For this review, take the finished solid that the model builds, in its own axes (mm). Round coordinates to 2 decimals unless told otherwise and drop trailing zeros. Order: outer loops, then holes, each group sorted by start corner. A loop starts at its lowest first (then second) coordinate and runs counter-clockwise, first axis right, second up. Notation, with made-up numbers: M -1,-21 L 29,-21 A27 cw 29,16 Z; hole C 9,88 d3. An arc over 180 degrees is marked long. Put each result on its own line as item: value.
from build123d import *

# Parameters (mm, degrees)
BOSS_EXTRUDE2_DEPTH   = 25.4
F_8_CLEARANCE_HOLE1_D = 4.191
FILLET1_R             = 2.54


with BuildPart() as part:
    # Sketch2 → Boss-Extrude2 (new body)
    with BuildSketch(Plane.XY):
        Polygon((92.922616299, 8.043671593), (48.599616303, 8.043671593), (48.599616303, 260.300358649), (92.922616299, 69.957537027), align=None)
    extrude(amount=BOSS_EXTRUDE2_DEPTH)

    # #8 Clearance Hole1 (through all)
    with Locations(Plane(origin=(0, 0, 0), x_dir=(-1, 0, 0), z_dir=(0, 0, -1))):
        with Locations((-80.22261633, 20.616671539), (-67.52261633, 20.616671539), (-54.82261633, 20.616671539)):
            Hole(F_8_CLEARANCE_HOLE1_D / 2)

    # Fillet1
    fillet1_edges = [part.edges().sort_by_distance(p)[0] for p in [
        (92.922616299, 39.00060431, 25.4),
        (70.761116301, 165.128947838, 25.4),
        (48.599616303, 134.172015121, 25.4),
        (70.761116301, 165.128947838, 0),
        (92.922616299, 39.00060431, 0),
        (70.761116301, 8.043671593, 0),
        (48.599616303, 134.172015121, 0),
        (70.761116301, 8.043671593, 25.4),
        (48.599616303, 260.300358649, 12.7),
        (92.922616299, 69.957537027, 12.7),
        (92.922616299, 8.043671593, 12.7),
        (48.599616303, 8.043671593, 12.7),
    ]]
    fillet(fillet1_edges, radius=FILLET1_R)


solid = part.part
(1) Insertion check: pin 1 Ø3.5 at (x, y) = (80.22, 20.62) entering from +Z; pin 2 Ø6.5 at (x, y) = (54.82, 20.62) entering from -Z; pin 3 Ø12 at (y, z) = (191.5, 12) entering from +X. Each pin has a flat end and moves straight along its axis. Give the tip position at first contact, or say it passes through.
A:
pin 1: passes through
pin 2: stops at z = 0
pin 3: stops at x = 66.02
(2) Draft analysis for pull direction X (two halves, no side actions). For faces 1 (the face through (48.6, 123, 13)), 2 (the face through (72.766, 153.152, 0.724)), 3 (the face through (78.13, 20.71, 12.88)), 4 (the face through (67, 101, 0)), state which applies: released by +X, released by -X, zero draft, split by the parting line, or undercut.
A:
face 1: released by -X
face 2: released by +X
face 3: undercut
face 4: zero draft
(3) Add section A-A on z = 6.75. Give the boundary of the cut face in (x, y).
A:
outline: M 48.6,10.58 A2.54 ccw 51.14,8.04 L 90.38,8.04 A2.54 ccw 92.92,10.58 L 92.92,69.67 A2.54 ccw 92.86,70.24 L 53.61,238.77 A2.54 ccw 48.6,238.19 Z; hole C 54.82,20.62 d4.19; hole C 67.52,20.62 d4.19; hole C 80.22,20.62 d4.19
(4) To check wall thickness, follow L1, parallel to X at y = 108, z = 18.25; L2, parallel to Z at x = 56, y = 224.5; L3, parallel to Z at x = 86, y = 91.5. State the ranges of each line that lie inside material, in increasing order.
A:
L1: x = 48.6 to 84.06
L2: z = 0.59 to 24.81
L3: z = 0.09 to 25.31
